from build123d import *

# Parameters (mm, degrees)
ESQUISSE1_R             = 1.5
BOSS_EXTRU_2_DEPTH      = 5
ENL_V_MAT_EXTRU_2_DEPTH = 2


with BuildPart() as part:
    # Esquisse1 → Boss.-Extru.2 (new body)
    with BuildSketch(Plane.XY):
        Polygon((22, -30.022213998), (-32, -30.022213998), (-32, -29.022213998), (-35, -29.022213998), (-35, -30.022213998), (-42, -30.022213998), (-52, -12.701705922), (-52, -5.701705922), (-51, -5.701705922), (-51, -2.701705922), (-52, -2.701705922), (-52, 8.475208614), (-51, 8.475208614), (-51, 11.475208614), (-52, 11.475208614), (-52, 18.475208614), (-42, 35.79571669), (-35, 35.79571669), (-35, 34.79571669), (-32, 34.79571669), (-32, 35.79571669), (22, 35.79571669), (22, 34.79571669), (25, 34.79571669), (25, 35.79571669), (32, 35.79571669), (42, 18.475208614), (42, 11.475208614), (41, 11.475208614), (41, 8.475208614), (42, 8.475208614), (42, -2.701705922), (41, -2.701705922), (41, -5.701705922), (42, -5.701705922), (42, -12.701705922), (32, -30.022213998), (25, -30.022213998), (25, -29.022213998), (22, -29.022213998), align=None)
        with Locations((17.5, 25.386751346)):
            Circle(ESQUISSE1_R, mode=Mode.SUBTRACT)
        with Locations((-27.5, 25.386751346)):
            Circle(ESQUISSE1_R, mode=Mode.SUBTRACT)
        with Locations((17.5, -19.613248654)):
            Circle(ESQUISSE1_R, mode=Mode.SUBTRACT)
        with Locations((-27.5, -19.613248654)):
            Circle(ESQUISSE1_R, mode=Mode.SUBTRACT)
        Polygon((-45, 8.475208614), (-45, -2.701705922), (-46, -2.701705922), (-46, -5.701705922), (-45, -5.701705922), (-45, -10.826061575), (-21.248711306, 2.886751346), (-45, 16.599564267), (-45, 11.475208614), (-46, 11.475208614), (-46, 8.475208614), align=None, mode=Mode.SUBTRACT)
        Polygon((35, 16.599564267), (11.248711306, 2.886751346), (35, -10.826061575), (35, -5.701705922), (36, -5.701705922), (36, -2.701705922), (35, -2.701705922), (35, 8.475208614), (36, 8.475208614), (36, 11.475208614), (35, 11.475208614), align=None, mode=Mode.SUBTRACT)
        Polygon((-37.958548116, -23.022213998), (-35, -23.022213998), (-35, -24.022213998), (-32, -24.022213998), (-32, -23.022213998), (-30.5, -23.022213998), (-30.5, -18.716019236), align=None, mode=Mode.SUBTRACT)
        Polygon((14.5, -23.022213998), (-5, -23.022213998), (-24.5, -23.022213998), (-24.5, -15.25191762), (-5, -3.993587371), (14.5, -15.25191762), align=None, mode=Mode.SUBTRACT)
        Polygon((-32, 29.79571669), (-32, 28.79571669), (-30.5, 28.79571669), (-30.5, 24.489521927), (-37.958548116, 28.79571669), (-35, 28.79571669), (-35, 29.79571669), align=None, mode=Mode.SUBTRACT)
        Polygon((27.958548116, 28.79571669), (20.5, 24.489521927), (20.5, 28.79571669), (22, 28.79571669), (22, 29.79571669), (25, 29.79571669), (25, 28.79571669), align=None, mode=Mode.SUBTRACT)
        Polygon((22, -24.022213998), (22, -23.022213998), (20.5, -23.022213998), (20.5, -18.716019236), (27.958548116, -23.022213998), (25, -23.022213998), (25, -24.022213998), align=None, mode=Mode.SUBTRACT)
        Polygon((-24.5, 28.79571669), (-24.5, 21.025420312), (-5, 9.767090063), (14.5, 21.025420312), (14.5, 28.79571669), (-5, 28.79571669), align=None, mode=Mode.SUBTRACT)
    extrude(amount=BOSS_EXTRU_2_DEPTH)

    # Esquisse4 → Enlèv. mat.-Extru.2 (cut)
    with BuildSketch(Plane(origin=(0, 0, 0), x_dir=(-1, 0, 0), z_dir=(0, 0, -1))):
        Polygon((-17.5, 23.029642358), (-15.458683737, 24.208196852), (-15.458683737, 26.56530584), (-17.5, 27.743860334), (-19.541316263, 26.56530584), (-19.541316263, 24.208196852), align=None)
        Polygon((29.541316263, 24.208196852), (27.5, 23.029642358), (25.458683737, 24.208196852), (25.458683737, 26.56530584), (27.5, 27.743860334), (29.541316263, 26.56530584), align=None)
        Polygon((27.5, -17.256139666), (25.458683737, -18.43469416), (25.458683737, -20.791803148), (27.5, -21.970357642), (29.541316263, -20.791803148), (29.541316263, -18.43469416), align=None)
        Polygon((-19.541316263, -18.43469416), (-17.5, -17.256139666), (-15.458683737, -18.43469416), (-15.458683737, -20.791803148), (-17.5, -21.970357642), (-19.541316263, -20.791803148), align=None)
    extrude(amount=-ENL_V_MAT_EXTRU_2_DEPTH, mode=Mode.SUBTRACT)


solid = part.part
Can you work these out from the model? Positions are in its coordinate system, mm. A direction names the side the tool comes from. Round coordinates to 2 decimals unless told otherwise and drop trailing zeros. Write each loop counter-clockwise with the first axis right and the second up, starting at its lowest first coordinate (ties: lowest second). Pieces come first, ordered by that corner, then holes. Notation, with made-up numbers: (48, 87) -> (88, 87) arc R17 ccw to (88, 112) -> close; hole circle Ø8 at (-4.75, 42.5). An arc over 180 degrees is marked (long way). One line per question, with ' | ' between items. Start each with the question number.
1) I'm going to push flat-ended pins straight in: P1, Ø0.5, axis at x = -45.5, z = 1.5, coming from the +Y side; P2, Ø1, axis at y = 26, z = 1, coming from the +X side; P3, Ø1.2, axis at x = 17, y = 25, coming from the -Z side; P4, Ø0.6, axis at y = -19.5, z = 1.5, coming from the -X side. Where does each tip first touch, or does it pass through?
2) Suppose I cut it at C-C on x = -12.5. Write out the boundary of the cut face in (y, z).
3) Suppose I cut it at A-A on x = 23. Write out the boundary of the cut face in (y, z), then the cut area to 3 significant figures.
4) On a 3-axis mill with a long thin cutter (end or side, diameter ignored), from which of +Z, -Z, +X, -X, +Y, -Y can I reach the whole of each face in a straight line? I mean faces 4 (the flat face through (37.07, -21.24, 2.46)), 5 (the flat face through (41, -4, 2)), 6 (the flat face through (16.494, 23.611, 0.986)), 7 (the flat face through (-5, -23.022, 2)). Say none if no direction works.
5) I need wall thicknesses on line 1 (Y direction, x = -13, z = 0.5); line 2 (X direction, y = 26, z = 1.3); line 3 (X direction, y = -10, z = 3). Which ranges of each line are inside material? Lowest first, please. Write a range as [from, to].
6) Suppose I cut it at D-D on z = 4.2. Count the separate pieces of the cut face and the enclosed holes in it, then the cut area to 3 significant figures.
7) If we mould it in two halves opening along Y, with no side actions, what happens to faces 1 (the flat face through (24, -29.022, 2)), 2 (the flat face through (28, 35.796, 2)), 3 (the flat face through (24.18, -20.84, 2.46))? For each: released by +Y, released by -Y, zero draft, split by the parting line, or undercut.
8) Suppose I cut it at B-B on y = 5. Write out the boundary of the cut face in (x, z), then the cut area to 3 significant figures.
Return value:
1) P1: stops at y = 30.17 | P2: stops at x = 37.94 | P3: passes through | P4: stops at x = -48.25
2) outline: (-30.02, 0) -> (-23.02, 0) -> (-23.02, 5) -> (-30.02, 5) -> close; (-8.32, 0) -> (14.1, 0) -> (14.1, 5) -> (-8.32, 5) -> close; (28.8, 0) -> (35.8, 0) -> (35.8, 5) -> (28.8, 5) -> close
3) outline: (-29.02, 0) -> (-24.02, 0) -> (-24.02, 5) -> (-29.02, 5) -> close; (-20.16, 0) -> (-3.9, 0) -> (-3.9, 5) -> (-20.16, 5) -> close; (9.67, 0) -> (25.93, 0) -> (25.93, 5) -> (9.67, 5) -> close; (29.8, 0) -> (34.8, 0) -> (34.8, 5) -> (29.8, 5) -> close | area: 213 mm2
4) face 4: +Z, -Z, +X, -Y | face 5: +Z, -Z, +X | face 6: -Z | face 7: +Z, -Z
5) line 1: y = [-30.02, -23.02], [-8.61, 14.39], [28.8, 35.8] | line 2: x = [-47.66, -33.12], [-30.5, -29.54], [-25.46, -24.5], [14.5, 15.46], [19.54, 20.5], [23.12, 37.66] | line 3: x = [-52, -45], [-43.57, -15.4], [5.4, 33.57], [35, 42]
6) separate pieces: 1 | enclosed holes: 12 | area: 4,000 mm2
7) face 1: released by -Y | face 2: released by +Y | face 3: undercut
8) outline: (-52, 0) -> (-45, 0) -> (-45, 5) -> (-52, 5) -> close; (-24.91, 0) -> (14.91, 0) -> (14.91, 5) -> (-24.91, 5) -> close; (35, 0) -> (42, 0) -> (42, 5) -> (35, 5) -> close | area: 269 mm2
